Autodesk Inventor part; units mm, degrees
ref_plane "YZ Plane" through (0, 0, 0) normal (1, 0, 0) x (0, 1, 0)
ref_plane "XZ Plane" through (0, 0, 0) normal (0, 1, 0) x (-1, 0, 0)
ref_plane "XY Plane" through (0, 0, 0) normal (0, 0, 1) x (1, 0, 0)
sketch "Sketch5" plane through (0, 0, 0) normal (0, 1, 0) x (-1, 0, 0)
  line L0 (56.5, 52.5) -> (-56.5, 52.5)
  line L1 (-56.5, 52.5) -> (-56.5, -52.5)
  line L2 (-56.5, -52.5) -> (56.5, -52.5)
  line L3 (56.5, -52.5) -> (56.5, 52.5)
  point P0 (0, 0)
  point P1 (56.5, 0)
  point P2 (0, 52.5)
  dimension "d8" = 113
  dimension "d9" = 105
extrude "Extrusion5" add sketch "Sketch5" along normal blind 107.5
sketch "Sketch8" plane through (0, 107.5, 0) normal (0, 1, 0) x (1, 0, 0)
  circle A0 centre (0, 27.5) radius 7
  circle A1 centre (0, -27.5) radius 7
  line L0 (-56.5, -52.5) -> (56.5, -52.5)
  line L1 (56.5, -52.5) -> (56.5, 52.5)
  line L2 (56.5, 52.5) -> (-56.5, 52.5)
  line L3 (-56.5, 52.5) -> (-56.5, -52.5)
  point P0 (0, 52.5)
  point P1 (0, -52.5)
  point P2 (56.5, 0)
  point P3 (-56.5, 0)
  point P4 (0, -52.5)
  dimension "d21" = 113
  dimension "d22" = 105
  dimension "d61" = 55
  dimension "d62" = 27.5
hole "Hole1" at (0, 107.5, 27.5) at (0, 107.5, -27.5) direction (0, -1, 0) diameter 9 end through all counterbore diameter 15 counterbore depth 45
sketch "Sketch9" plane through (-56.5, 0, 52.5) normal (0, 0, 1) x (1, 0, 0)
  line L0 (0, 0) -> (0, 107.5)
  circle A0 centre (15, 93.75) radius 4
  circle A1 centre (15, 53.75) radius 4
  circle A2 centre (15, 13.75) radius 4
  point P0 (113, 0)
  point P1 (113, 107.5)
  point P2 (56.5, 0)
  point P3 (0, 53.75)
  dimension "d36" = 107.5
  dimension "d37" = 40
  dimension "d38" = 40
  dimension "d40" = 8
  dimension "d41" = 15
hole "Hole2" at (-41.5, 93.75, 52.5) at (-41.5, 53.75, 52.5) at (-41.5, 13.75, 52.5) direction (0, 0, -1) diameter 6.647 depth 15 tip angle 118
sketch "Sketch10" plane through (56.5, 0, -52.5) normal (0, 0, -1) x (-1, 0, 0)
  circle A0 centre (98, 93.75) radius 4
  circle A1 centre (98, 53.75) radius 4
  circle A2 centre (98, 13.75) radius 4
  circle A3 centre (98, 53.75) radius 3.3235
  circle A4 centre (98, 13.75) radius 3.3235
  circle A5 centre (98, 93.75) radius 3.3235
  dimension "d52" = 8
hole "Hole3" at (-41.5, 93.75, -52.5) at (-41.5, 53.75, -52.5) at (-41.5, 13.75, -52.5) direction (0, 0, 1) diameter 6.647 depth 15 tip angle 118
sketch "Sketch11" plane through (0, 107.5, 0) normal (0, 1, 0) x (1, 0, 0)
  line L0 (-56.5, 52.5) -> (-56.5, -52.5)
  circle A0 centre (-46.5, -27.5) radius 4
  circle A1 centre (-46.5, 27.5) radius 4
  point P0 (0, 0)
  dimension "d63" = 55
  dimension "d64" = 10
  dimension "d65" = 8
  dimension "d73" = 27.5
hole "Hole4" at (-46.5, 107.5, 27.5) at (-46.5, 107.5, -27.5) direction (0, -1, 0) diameter 4.134 depth 15 tip angle 118
chamfer "Chamfer2" distance 1 angle 45 12 edges at (56.5, 53.75, -52.5) (56.5, 53.75, 52.5) (-56.5, 53.75, 52.5) (-56.5, 53.75, -52.5) (0, 107.5, -52.5) (-56.5, 107.5, 0) (0, 107.5, 52.5) (56.5, 107.5, 0) (0, 0, -52.5) (-56.5, 0, 0) (0, 0, 52.5) (56.5, 0, 0)
equation "\"d38\" = d37"
properties part number "BC-10002" material "Aço Carbono AISI 1006"
Geometry check sheet. Reference: the model listing, model coordinates, mm. A direction names the side the tool comes from. Coordinates: 2 decimals unless noted, no trailing zeros. Loops run counter-clockwise (first coordinate to the right, second up) from the corner with the lowest first, then second, coordinate; pieces in that order, holes last. Notation, with made-up numbers: (-26, 83) - (13, 83) arc R28 ccw to (13, 121) - close; hole circle Ø6 at (-7.5, 62). An arc over 180 degrees is marked (long way). One line per item, written item: value. Start each with the question number.
(1) Depth check by flat-ended pin: P1, Ø10.5, axis at x = 0, z = -27.5, coming from the +Y side; P2, Ø6, axis at x = -41.5, y = 53.75, coming from the +Z side. Enter the tip coordinate at first touch or a pass-through.
(2) Cross-section at B-B on y = 66. Enter the section's corners in (x, z).
(3) Cross-section at A-A on x = 0. Enter the section's corners in (y, z), plus the area to 3 significant figures.
(4) Material ranges on line 1 (Z direction, x = 0, y = 87); line 2 (Y direction, x = -41.5, z = -44); line 3 (Y direction, x = -41, z = 48), recorded low to high. Write a range as [from, to].
(5) Tool access check on faces 3 (the cylindrical face through (-39.48, 56.39, 44.9)), 4 (the cylindrical face through (-41.65, 90.43, -44.9)), 5 (the cylindrical face through (0, 85, 20)). Record the directions out of +Z, -Z, +X, -X, +Y, -Y that give a thin tool (end or side, any length) a straight path to the whole face; none if there is none.
(6) Mould release check, pull along X, two halves, no side actions. Record for faces 1 (the flat face through (-1, 53, 52.5)), 2 (the cylindrical face through (0, 85, -35)): released by +X, released by -X, zero draft, split by the parting line, or undercut.
Results below:
1. P1: stops at y = 62.5
1. P2: stops at z = 37.31
2. outline: (-56.5, -51.5) - (-55.5, -52.5) - (55.5, -52.5) - (56.5, -51.5) - (56.5, 51.5) - (55.5, 52.5) - (-55.5, 52.5) - (-56.5, 51.5) - close; hole circle Ø15 at (0, -27.5); hole circle Ø15 at (0, 27.5)
3. outline: (0, -51.5) - (1, -52.5) - (106.5, -52.5) - (107.5, -51.5) - (107.5, -35) - (62.5, -35) - (62.5, -32) - (0, -32) - close; (0, -23) - (62.5, -23) - (62.5, -20) - (107.5, -20) - (107.5, 20) - (62.5, 20) - (62.5, 23) - (0, 23) - close; (0, 32) - (62.5, 32) - (62.5, 35) - (107.5, 35) - (107.5, 51.5) - (106.5, 52.5) - (1, 52.5) - (0, 51.5) - close
3. area: 8,810 mm2
4. line 1: z = [-52.5, -35], [-20, 20], [35, 52.5]
4. line 2: y = [0, 10.43], [17.07, 50.43], [57.07, 90.43], [97.07, 107.5]
4. line 3: y = [0, 10.46], [17.04, 50.46], [57.04, 90.46], [97.04, 107.5]
5. face 3: +Z
5. face 4: -Z
5. face 5: +Y
6. face 1: zero draft
6. face 2: undercut
